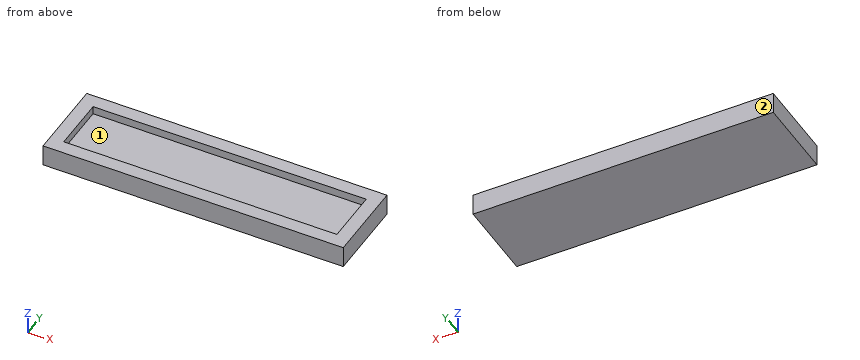
```python
from build123d import *

# Parameters (mm, degrees)
F0_W     = 56.261
F0_H     = 15.4178
F0_W_2   = 51.181
F0_H_2   = 10.3378
F1_DEPTH = 1.27
F2_DEPTH = 2.794


# Not quite as in the source:
# - a feature names something its author has since deleted; it is built from what else it names


with BuildPart() as f1:
    # F0 (on Top) → F1 (new body, symmetric)
    with BuildSketch(Plane.XY):
        Rectangle(F0_W, F0_H)
        Rectangle(F0_W_2, F0_H_2, mode=Mode.SUBTRACT)
        Rectangle(F0_W_2, F0_H_2)
    extrude(amount=F1_DEPTH, both=True)

    # F0 (on Top) → F2 (join)
    with BuildSketch(Plane.XY):
        Rectangle(F0_W, F0_H)
        Rectangle(F0_W_2, F0_H_2, mode=Mode.SUBTRACT)
    extrude(amount=F2_DEPTH)


solid = f1.part
```
CAD build for the part. Positions are in the model's coordinates, mm. Face numbers are marked on the shaded views. Round coordinates to 2 decimals unless told otherwise and drop trailing zeros. Loops run counter-clockwise (first coordinate to the right, second up) from the corner with the lowest first, then second, coordinate; pieces in that order, holes last. Notation, with made-up numbers: M -13.5,-7 L 23.5,-7 A6 cw 23.5,-3 Z; hole C 15,-30.5 d10. An arc over 180 degrees is marked long. Return JSON: item names as keys, results as strings. Group by question number.
(1) Saw through at B-B, the plane x = -19.5. List the corners of the cut face in (y, z), and give its area (3 significant figures).
(2) Mould opens along X. For the marked faces 1 and 2 say: +X half, -X half, draft (parallel to the pull), parting line (faces both ways), or undercut.
(3) Drop a flat-ended pin along its axis: P1, Ø5, axis at x = -2, y = -1, coming from the +Z side. Give the stop position or say it passes through.
(4) Saw through at C-C, the plane y = 2. List the corners of the cut face in (x, z).
(5) Wall check: probe 1 along Y at (x, z) = (-3, 2.65); probe 2 along Z at (x, y) = (-22, -2.75); probe 3 along X at (y, z) = (3.5, 2.35). Give the ranges that are in metal, low to high. Write a range as [from, to].
(6) Saw through at A-A, the plane z = 2.1. List the corners of the cut face in (x, y), and give its area (3 significant figures).
Answer list:
{
 "1": {"outline": "M -7.71,-1.27 L 7.71,-1.27 L 7.71,2.79 L 5.17,2.79 L 5.17,1.27 L -5.17,1.27 L -5.17,2.79 L -7.71,2.79 Z", "area": "46.9 mm2"},
 "2": {"face 1": "undercut", "face 2": "draft"},
 "3": {"P1": "z = 1.27"},
 "4": {"outline": "M -28.13,-1.27 L 28.13,-1.27 L 28.13,2.79 L 25.59,2.79 L 25.59,1.27 L -25.59,1.27 L -25.59,2.79 L -28.13,2.79 Z"},
 "5": {"probe 1": "[-7.71, -5.17], [5.17, 7.71]", "probe 2": "[-1.27, 1.27]", "probe 3": "[-28.13, -25.59], [25.59, 28.13]"},
 "6": {"outline": "M -28.13,-7.71 L 28.13,-7.71 L 28.13,7.71 L -28.13,7.71 Z; hole M -25.59,-5.17 L 25.59,-5.17 L 25.59,5.17 L -25.59,5.17 Z", "area": "338 mm2"}
}
